```python
from build123d import *

# Parameters (mm, degrees)
SKETCH1_R           = 8
BOSS_EXTRUDE1_DEPTH = 4
SKETCH2_R           = 2.75
BOSS_EXTRUDE2_DEPTH = 4
BOSS_EXTRUDE3_DEPTH = 42


with BuildPart() as part:
    # Sketch1 → Boss-Extrude1 (new body)
    with BuildSketch(Plane.XY):
        with BuildLine():
            Line((0, 0), (9.971912122, 21.384834556))
            ThreePointArc((9.971912122, 21.384834556), (21, 28), (32.028087878, 21.384834556))
            Line((32.028087878, 21.384834556), (42, 0))
            Line((42, 0), (0, 0))
        make_face()
        with Locations((21, 15.5)):
            Circle(SKETCH1_R, mode=Mode.SUBTRACT)
    extrude(amount=BOSS_EXTRUDE1_DEPTH)



with BuildPart() as body_2:
    # Sketch2 → Boss-Extrude2 (new body)
    with BuildSketch(Plane(origin=(0, 0, 0), x_dir=(-1, 0, 0), z_dir=(0, -1, 0))):
        with BuildLine():
            Line((0, -4), (0, -18))
            ThreePointArc((0, -18), (-0.585786438, -19.414213562), (-2, -20))
            Line((-2, -20), (-40, -20))
            ThreePointArc((-40, -20), (-41.414213562, -19.414213562), (-42, -18))
            Line((-42, -18), (-42, -4))
            Line((-42, -4), (0, -4))
        make_face()
        with Locations(Location((-37, -14, 0), (0, 0, 90))):
            Circle(SKETCH2_R, mode=Mode.SUBTRACT)
        with Locations(Location((-5, -14, 0), (0, 0, 90))):
            Circle(SKETCH2_R, mode=Mode.SUBTRACT)
    extrude(amount=BOSS_EXTRUDE2_DEPTH)


with BuildPart() as part_1:
    add(part.part)

    add(body_2.part)  # Boss-Extrude3 merges body 2
    # Sketch3 → Boss-Extrude3 (add)
    with BuildSketch(Plane.ZY):
        with BuildLine():
            Line((4, 0), (0, 0))
            ThreePointArc((0, 0), (1.171572875, -2.828427125), (4, -4))
            Line((4, -4), (4, 0))
        make_face()
    extrude(amount=-BOSS_EXTRUDE3_DEPTH)


solid = part_1.part
```
Verification items for the finished model (mm, model axes). A direction names the side the tool comes from. Coordinates: 2 decimals unless noted, no trailing zeros. Loops run counter-clockwise (first coordinate to the right, second up) from the corner with the lowest first, then second, coordinate; pieces in that order, holes last. Notation, with made-up numbers: (16, 1) -> (20, 1) arc R19 cw to (20, 7) -> close; hole circle Ø9 at (-11, 35). An arc over 180 degrees is marked (long way). Put each result on its own line as item: value.
1. Section check C-C, the plane y = 20. Record the boundary of the cut face in (x, z).
Result set:
outline: (9.33, 0) -> (14.39, 0) -> (14.39, 4) -> (9.33, 4) -> close; (27.61, 0) -> (32.67, 0) -> (32.67, 4) -> (27.61, 4) -> close
2. Section check D-D, the plane x = 5. Record the boundary of the cut face in (y, z).
Result set:
outline: (-4, 4) arc R4 ccw to (0, 0) -> (10.72, 0) -> (10.72, 4) -> (0, 4) -> (0, 11.25) -> (-4, 11.25) -> close; (-4, 16.75) -> (0, 16.75) -> (0, 20) -> (-4, 20) -> close
3. Section check B-B, the plane x = 21. Record the boundary of the cut face in (y, z), then the cut area to 3 significant figures.
Result set:
outline: (-4, 4) arc R4 ccw to (0, 0) -> (7.5, 0) -> (7.5, 4) -> (0, 4) -> (0, 20) -> (-4, 20) -> close; (23.5, 0) -> (28, 0) -> (28, 4) -> (23.5, 4) -> close
area: 125 mm^2
4. Mould release check, pull along Y, two halves, no side actions. Record for faces 3 (the face through (5.121, -1.972, 16.747)), 4 (the face through (20.706, -2.797, 1.141)), 5 (the face through (21, 28, 2)), 6 (the face through (14.651, 10.632, 1.972)): pulls with the +Y half, pulls with the -Y half, needs draft (parallel to the pull), parting line crosses it, or undercut.
Result set:
face 3: needs draft
face 4: pulls with the -Y half
face 5: pulls with the +Y half
face 6: undercut
5. Gauge pin test, flat ends, axial feed: P1, Ø1, axis at x = 5.5, y = 4, coming from the +Z side; P2, Ø12, axis at y = 10, z = 7, coming from the -X side. Record the tip position at first contact, or that the pin passes through.
Result set:
P1: stops at z = 4
P2: stops at x = 2.24
6. Thickness scan on line 1 (X direction, y = -2.35, z = 14); line 2 (Z direction, x = 10, y = 12); line 3 (Y direction, x = 17, z = 9.25). Record the ranges inside material, lowest first.
Result set:
line 1: x = 0 to 2.25, 7.75 to 34.25, 39.75 to 42
line 2: z = 0 to 4
line 3: y = -4 to 0
7. Tool access check on faces 1 (the face through (39.727, -1.972, 14.358)), 2 (the face through (21, 0, 12)). Record the directions out of +Z, -Z, +X, -X, +Y, -Y that give a thin tool (end or side, any length) a straight path to the whole face; none if there is none.
Result set:
face 1: +Y, -Y
face 2: +Z, +X, -X, +Y
8. Section check A-A, the plane z = 14. Record the boundary of the cut face in (x, y).
Result set:
outline: (0, -4) -> (2.25, -4) -> (2.25, 0) -> (0, 0) -> close; (7.75, -4) -> (34.25, -4) -> (34.25, 0) -> (7.75, 0) -> close; (39.75, -4) -> (42, -4) -> (42, 0) -> (39.75, 0) -> close
